The figure shows three views and two pictorial views of one solid part (mm, origin at its lowest corner). Answer the questions. A direction names the side the tool comes from. Coordinates: 2 decimals unless noted, no trailing zeros. Write each loop counter-clockwise with the first axis right and the second up, starting at its lowest first coordinate (ties: lowest second). Pieces come first, ordered by that corner, then holes.
Item 1: Section C-C (y = 165) is taken. Give the vertices of the cut face in (x, z).
Item 2: Section B-B (z = 130) is taken. Give the vertices of the cut face in (x, y), then the cut area to 3 significant figures.
Item 3: A tool of negligible diameter and unlimited length cuts with its end or side. For the marked faces 1, 2 and 3, from which of +Z, -Z, +X, -X, +Y, -Y can it reach the whole face along a straight path? Write none if from no direction.
Item 4: Straight lines are drawn through the part: probe 1 along Z at (x, y) = (180.5, 100); probe 2 along Y at (x, z) = (133, 130.5); probe 3 along Z at (x, y) = (279, 97.5). For each, find the intervals that lie inside material, in ascending order.
Item 5: Section A-A (y = 100) is taken. Give the vertices of the cut face in (x, z).
Item 6: Each of these flat-tipped pins is pushed along its axis until it touches: P1, Ø12, axis at x = 77.5, y = 44, coming from the +Z side; P2, Ø1, axis at y = 100.5, z = 59.5, coming from the -X side; P3, Ø12, axis at x = 86, z = 60.5, coming from the -Y side; P4, Ø12, axis at y = 139.5, z = 194, coming from the +X side. Where does it stop, or does it pass through?
Item 7: Section D-D (z = 218.5) is taken. Give the vertices of the cut face in (x, y).
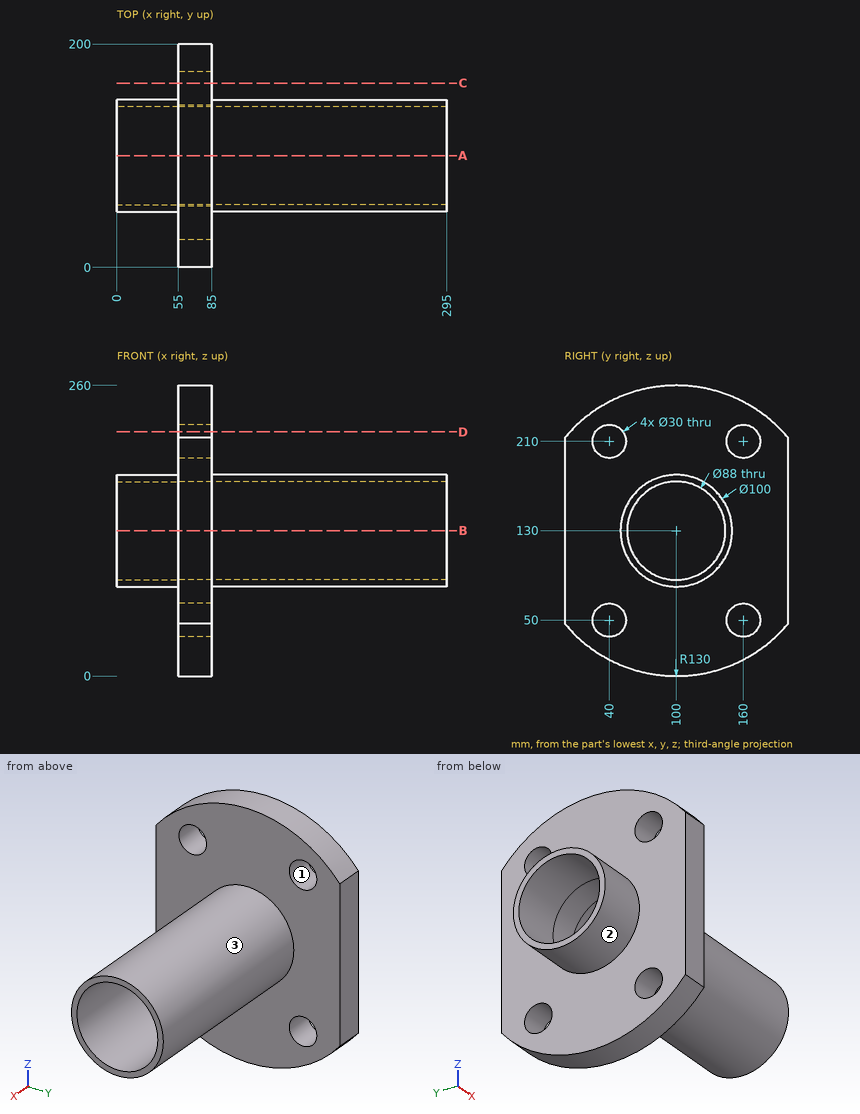
Established:
1. outline: (55, 17.42) - (85, 17.42) - (85, 35.86) - (55, 35.86) - close; (55, 64.14) - (85, 64.14) - (85, 195.86) - (55, 195.86) - close; (55, 224.14) - (85, 224.14) - (85, 242.58) - (55, 242.58) - close
2. outline: (0, 50) - (55, 50) - (55, 0) - (85, 0) - (85, 50) - (295, 50) - (295, 56) - (0, 56) - close; (0, 144) - (295, 144) - (295, 150) - (85, 150) - (85, 200) - (55, 200) - (55, 150) - (0, 150) - close
2. area: 6,540 mm2
3. face 1: +X, -X
3. face 2: -X
3. face 3: +X
4. probe 1: z = 80 to 86, 174 to 180
4. probe 2: y = 50 to 56, 144 to 150
4. probe 3: z = 80.06 to 86.07, 173.93 to 179.94
5. outline: (0, 80) - (55, 80) - (55, 0) - (85, 0) - (85, 80) - (295, 80) - (295, 86) - (0, 86) - close; (0, 174) - (295, 174) - (295, 180) - (85, 180) - (85, 260) - (55, 260) - (55, 180) - (0, 180) - close
6. P1: stops at z = 250
6. P2: stops at x = 55
6. P3: stops at y = 0
6. P4: stops at x = 85
7. outline: (55, 4.78) - (85, 4.78) - (85, 27.64) - (55, 27.64) - close; (55, 52.36) - (85, 52.36) - (85, 147.64) - (55, 147.64) - close; (55, 172.36) - (85, 172.36) - (85, 195.22) - (55, 195.22) - close
